from build123d import *

# Parameters (mm, degrees)
SKETCH1_W           = 55
SKETCH1_H           = 55
SKETCH1_R           = 15
BOSS_EXTRUDE3_DEPTH = 9
BOSS_EXTRUDE4_DEPTH = 34
CUT_EXTRUDE1_REACH  = 60.644
SKETCH6_R           = 2.5


with BuildPart() as part:
    # Sketch1 → Boss-Extrude3 (new body)
    with BuildSketch(Plane(origin=(0, 0, 0), x_dir=(1, 0, 0), z_dir=(0, 1, 0))):
        with Locations((-0.141805914, 1.240284381)):
            Rectangle(SKETCH1_W, SKETCH1_H)
        with Locations(Location((-0.141805914, 1.240284381, 0), (0, 0, 270))):
            Circle(SKETCH1_R, mode=Mode.SUBTRACT)
    extrude(amount=BOSS_EXTRUDE3_DEPTH)

    # Sketch5 → Boss-Extrude4 (add)
    with BuildSketch(Plane(origin=(0, 9, 0), x_dir=(1, 0, 0), z_dir=(0, 1, 0))):
        with BuildLine():
            ThreePointArc((14.858194086, 1.240284381), (-0.141805914, -13.759715619), (-15.141805914, 1.240284381))
            Line((-15.141805914, 1.240284381), (-15.141805914, 28.740284381))
            Line((-15.141805914, 28.740284381), (-27.641805914, 28.740284381))
            Line((-27.641805914, 28.740284381), (-27.641805914, -26.259715619))
            Line((-27.641805914, -26.259715619), (27.358194086, -26.259715619))
            Line((27.358194086, -26.259715619), (27.358194086, 28.740284381))
            Line((27.358194086, 28.740284381), (14.858194086, 28.740284381))
            Line((14.858194086, 28.740284381), (14.858194086, 1.240284381))
        make_face()
    extrude(amount=BOSS_EXTRUDE4_DEPTH)

    # Sketch6 → Cut-Extrude1 (cut, up to next)
    with BuildSketch(Plane.XZ, mode=Mode.PRIVATE) as cut_extrude1_sk1:
        with Locations(Location((-23.711805914, 22.329715619, 0), (0, 0, 270))):
            Circle(SKETCH6_R)
    cut_extrude1_tool1 = extrude(cut_extrude1_sk1.sketch, amount=-CUT_EXTRUDE1_REACH, mode=Mode.PRIVATE) & part.part
    # Sketch6 → Cut-Extrude1 (cut, up to next)
    with BuildSketch(Plane.XZ, mode=Mode.PRIVATE) as cut_extrude1_sk2:
        with Locations(Location((23.428194086, 22.329715619, 0), (0, 0, 270))):
            Circle(SKETCH6_R)
    cut_extrude1_tool2 = extrude(cut_extrude1_sk2.sketch, amount=-CUT_EXTRUDE1_REACH, mode=Mode.PRIVATE) & part.part
    # Sketch6 → Cut-Extrude1 (cut, up to next)
    with BuildSketch(Plane.XZ, mode=Mode.PRIVATE) as cut_extrude1_sk3:
        with Locations(Location((-23.711805914, -24.810284381, 0), (0, 0, 270))):
            Circle(SKETCH6_R)
    cut_extrude1_tool3 = extrude(cut_extrude1_sk3.sketch, amount=-CUT_EXTRUDE1_REACH, mode=Mode.PRIVATE) & part.part
    # Sketch6 → Cut-Extrude1 (cut, up to next)
    with BuildSketch(Plane.XZ, mode=Mode.PRIVATE) as cut_extrude1_sk4:
        with Locations(Location((23.428194086, -24.810284381, 0), (0, 0, 270))):
            Circle(SKETCH6_R)
    cut_extrude1_tool4 = extrude(cut_extrude1_sk4.sketch, amount=-CUT_EXTRUDE1_REACH, mode=Mode.PRIVATE) & part.part
    add(cut_extrude1_tool1.solids().sort_by_distance((-23.711806, 0, 22.329716))[0], mode=Mode.SUBTRACT)
    add(cut_extrude1_tool2.solids().sort_by_distance((23.428194, 0, 22.329716))[0], mode=Mode.SUBTRACT)
    add(cut_extrude1_tool3.solids().sort_by_distance((-23.711806, 0, -24.810284))[0], mode=Mode.SUBTRACT)
    add(cut_extrude1_tool4.solids().sort_by_distance((23.428194, 0, -24.810284))[0], mode=Mode.SUBTRACT)


solid = part.part
Geometry check sheet. Reference: the model listing, model coordinates, mm. A direction names the side the tool comes from. Give positions to 0.01 mm unless a question says otherwise; leave off trailing zeros. Order: outer loops, then holes, each group sorted by start corner. A loop starts at its lowest first (then second) coordinate and runs counter-clockwise, first axis right, second up. Notation, with made-up numbers: M 2,4 L 55,4 A13 ccw 55,20 Z; hole C 42,49.25 d11. An arc over 180 degrees is marked long. Use a Markdown table: item, result.
Item 1: Material ranges on line 1 along X through (y, z) = (22, -2); line 2 along X through (y, z) = (16, 21.5); line 3 along X through (y, z) = (5, 24), recorded low to high.
Answers follow:
| item | result |
|---|---|
| line 1 | x = -27.64 to -15.14, 14.86 to 27.36 |
| line 2 | x = -27.64 to -26.07, -21.35 to 21.07, 25.79 to 27.36 |
| line 3 | x = -27.64 to -25.57, -21.85 to 21.57, 25.29 to 27.36 |
Item 2: Section check B-B (z = -15.5). Record the cut outline in (x, y).
Answers follow:
| item | result |
|---|---|
| outline | M -27.64,0 L -4.8,0 L -4.8,9 L -15.14,9 L -15.14,43 L -27.64,43 Z; M 4.51,0 L 27.36,0 L 27.36,43 L 14.86,43 L 14.86,9 L 4.51,9 Z |
Item 3: Section check C-C (z = 21). Record the cut outline in (x, y).
Answers follow:
| item | result |
|---|---|
| outline | M -27.64,0 L -25.83,0 L -25.83,43 L -27.64,43 Z; M -21.59,0 L 21.31,0 L 21.31,43 L -21.59,43 Z; M 25.55,0 L 27.36,0 L 27.36,43 L 25.55,43 Z |
Item 4: Section check D-D (y = 12). Record the cut outline in (x, z).
Answers follow:
| item | result |
|---|---|
| outline | M -27.64,-28.74 L -15.14,-28.74 L -15.14,-1.24 A15 cw 14.86,-1.24 L 14.86,-28.74 L 27.36,-28.74 L 27.36,26.26 L -27.64,26.26 Z; hole C -23.71,-24.81 d5; hole C -23.71,22.33 d5; hole C 23.43,-24.81 d5; hole C 23.43,22.33 d5 |
Item 5: Tool access check on faces 1 (the flat face through (-13, 0, 11)), 2 (the flat face through (14.858, 26, -15)). Record the directions out of +Z, -Z, +X, -X, +Y, -Y that give a thin tool (end or side, any length) a straight path to the whole face; none if there is none.
Answers follow:
| item | result |
|---|---|
| face 1 | +Z, -Z, +X, -X, -Y |
| face 2 | -Z, +Y |
Item 6: Draft check along Z on faces 3 (the flat face through (0, 9, -21)), 4 (the cylindrical face through (-21.6, 21.2, -26.15)), 5 (the cylindrical face through (24.179, 21.199, 19.945)). Enter one of: +Z half, -Z half, draft (parallel to the pull), parting line (faces both ways), or undercut.
Answers follow:
| item | result |
|---|---|
| face 3 | draft |
| face 4 | undercut |
| face 5 | undercut |
Item 7: Section check A-A (x = 2.5). Record the cut outline in (y, z), and give its area (3 significant figures).
Answers follow:
| item | result |
|---|---|
| outline | M 0,-28.74 L 9,-28.74 L 9,-16.01 L 0,-16.01 Z; M 0,13.53 L 43,13.53 L 43,26.26 L 0,26.26 Z |
| area | 662 mm2 |
Item 8: Depth check by flat-ended pin: P1, Ø24, axis at x = -0.14, z = -1.24, coming from the +Y side; P2, Ø5, axis at x = -2, y = 23.5, coming from the -Z side. Enter the tip coordinate at first touch or a pass-through.
Answers follow:
| item | result |
|---|---|
| P1 | passes through |
| P2 | stops at z = 13.11 |
